The listing builds one solid part. Answer for the finished solid, in the listing's coordinates (mm). Face numbers are marked on the shaded views. A direction names the side the tool comes from. Round coordinates to 2 decimals unless told otherwise and drop trailing zeros. Write each loop counter-clockwise with the first axis right and the second up, starting at its lowest first coordinate (ties: lowest second). Pieces come first, ordered by that corner, then holes.
from build123d import *
from build123d.topology import SkipClean

# Parameters (mm, degrees)
SKETCH1_W                      = 4.2
SKETCH1_H                      = 2.4
F_0_8_0_8_DIAMETER_HOLE1_D     = 0.8
SKETCH6_R                      = 3.2
BOSS_EXTRUDE1_DEPTH            = 0.8
BOSS_EXTRUDE2_DEPTH            = 3
CUT_EXTRUDE1_DEPTH             = 2.2
BOSS_EXTRUDE3_DEPTH            = 2.2
BOSS_EXTRUDE4_DEPTH            = 0.8
BOSS_EXTRUDE5_START            = 1.6
SKETCH11_R                     = 2.4
BOSS_EXTRUDE5_DEPTH            = 1.6
SKETCH16_W                     = 7.2
SKETCH16_H                     = 1.6
F_3_2_3_2_DIAMETER_HOLE1_D     = 3.2
F_3_2_3_2_DIAMETER_HOLE1_DEPTH = 1.6


with BuildPart() as part:
    # Sketch1 → Revolve1 (revolve)
    with BuildSketch(Plane.XY):
        with Locations((-2.9, 1.2)):
            Rectangle(SKETCH1_W, SKETCH1_H)
    revolve(axis=Axis((-5, 0, 0), (1, 0, 0)))

    # Ø0.8 (0.8) Diameter Hole1 (through all)
    with Locations(Plane(origin=(-5, 0, -2.4), x_dir=(0, -1, 0), z_dir=(0, 0, -1))):
        with Locations((0, 0)):
            Hole(F_0_8_0_8_DIAMETER_HOLE1_D / 2)

    # Sketch6 → Boss-Extrude1 (add)
    with BuildSketch(Plane.ZY.offset(0.8)):
        Circle(SKETCH6_R)
    extrude(amount=-BOSS_EXTRUDE1_DEPTH)

    # Sketch7 → Boss-Extrude2 (add)
    with BuildSketch(Plane.ZY.offset(5)):
        with BuildLine():
            Line((-2.569046516, -0.4), (2.569046516, -0.4))
            ThreePointArc((2.569046516, -0.4), (0, -2.6), (-2.569046516, -0.4))
        make_face()
    extrude(amount=BOSS_EXTRUDE2_DEPTH)

    # Sketch8 → Cut-Extrude1 (cut)
    with SkipClean():  # the faces are left unmerged after this step: merging them gives an invalid solid
        with BuildSketch(Plane(origin=(-5, 0, 0), x_dir=(0, 0, -1), z_dir=(1, 0, 0))):
            with BuildLine():
                Line((2.569046516, -0.4), (2.366431913, -0.4))
                ThreePointArc((2.366431913, -0.4), (0, -2.4), (-2.366431913, -0.4))
                Line((-2.366431913, -0.4), (-2.569046516, -0.4))
                ThreePointArc((-2.569046516, -0.4), (0, -2.6), (2.569046516, -0.4))
            make_face()
        extrude(amount=-CUT_EXTRUDE1_DEPTH, mode=Mode.SUBTRACT)

    # Sketch9 → Boss-Extrude3 (add)
    with SkipClean():  # the faces are left unmerged after this step: merging them gives an invalid solid
        with BuildSketch(Plane.ZY.offset(5)):
            with BuildLine():
                Line((2.366431913, 0.4), (-2.366431913, 0.4))
                ThreePointArc((-2.366431913, 0.4), (0, 2.4), (2.366431913, 0.4))
            make_face()
        extrude(amount=BOSS_EXTRUDE3_DEPTH)

    # Sketch10 → Boss-Extrude4 (add)
    with SkipClean():  # the faces are left unmerged after this step: merging them gives an invalid solid
        with BuildSketch(Plane.ZY.offset(7.2)):
            with BuildLine():
                Line((2.569046516, 0.4), (-2.569046516, 0.4))
                ThreePointArc((-2.569046516, 0.4), (0, 2.6), (2.569046516, 0.4))
            make_face()
        extrude(amount=BOSS_EXTRUDE4_DEPTH)

    # Sketch11 → Boss-Extrude5 (add)
    with SkipClean():  # the faces are left unmerged after this step: merging them gives an invalid solid
        with BuildSketch(Plane(origin=(0, 0, 0), x_dir=(0, 0, -1), z_dir=(1, 0, 0)).offset(BOSS_EXTRUDE5_START)):
            with Locations(Location((0, 0, 0), (0, 0, 90))):
                Circle(SKETCH11_R)
        extrude(amount=-BOSS_EXTRUDE5_DEPTH)

    # Sketch16 → Cut-Revolve1 (revolve, cut)
    with SkipClean():  # the faces are left unmerged after this step: merging them gives an invalid solid
        with BuildSketch(Plane(origin=(0, 0, 0), x_dir=(-1, 0, 0), z_dir=(0, 0, -1)), mode=Mode.PRIVATE) as cut_revolve1_sk:
            with Locations((4.4, 0.8)):
                Rectangle(SKETCH16_W, SKETCH16_H)
        revolve(cut_revolve1_sk.sketch.rotate(Axis((-0.8, 0, 0), (-1, 0, 0)), 270), axis=Axis((-0.8, 0, 0), (-1, 0, 0)), mode=Mode.SUBTRACT)

    # Ø3.2 (3.2) Diameter Hole1
    with Locations(Plane(origin=(1.6, 0, 0), x_dir=(0, 0, -1), z_dir=(1, 0, 0))):
        with Locations((0, 0)):
            Hole(F_3_2_3_2_DIAMETER_HOLE1_D / 2, depth=F_3_2_3_2_DIAMETER_HOLE1_DEPTH)


solid = part.part
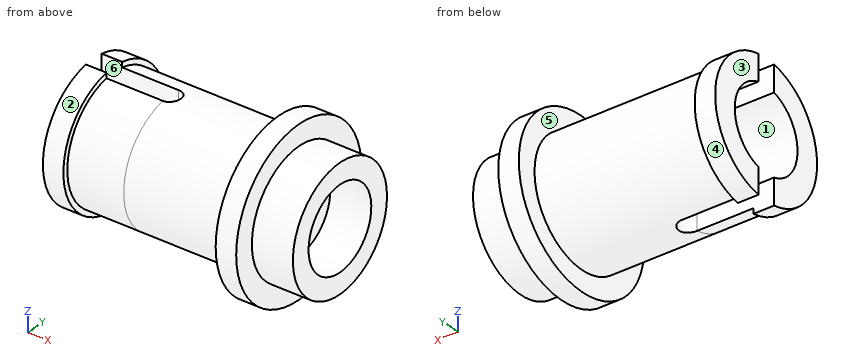
1. Given pin 1 (0.5 mm diameter, centred on x = -6.5, z = 2, fed in from +Y); pin 2 (1 mm diameter, centred on y = 0, z = -0.5, fed in from +X); pin 3 (0.8 mm diameter, centred on x = -6.5, z = 2, fed in from -Y), each flat-ended and moving along its own axis, determine where each tip first touches the part or whether it passes through.
Geometry says:
pin 1: stops at y = 1.64
pin 2: stops at x = 0
pin 3: stops at y = -1.79
2. Section A-A on x = -6 is taken. Determine the outline of the cut face in (y, z), plus the area to 3 significant figures.
Geometry says:
outline: (-0.4, -2.37) - (-0.4, -1.55) arc R1.6 cw to (-0.4, 1.55) - (-0.4, 2.37) arc R2.4 ccw to start; (0.4, -2.37) arc R2.4 ccw to (0.4, 2.37) - (0.4, 1.55) arc R1.6 cw to (0.4, -1.55) - close
area: 8.76 mm2
3. A tool of negligible diameter and unlimited length cuts with its end or side. For the marked faces 4, 5 and 6, from which of +Z, -Z, +X, -X, +Y, -Y can it reach the whole face along a straight path? Write none if from no direction.
Geometry says:
face 4: -X, +Y
face 5: none
face 6: +Z, -Z, -X
4. Section C-C on y = 0 is taken. Determine the outline of the cut face in (x, z).
Geometry says:
outline: (-4.6, -2.4) - (-0.8, -2.4) - (-0.8, -3.2) - (0, -3.2) - (0, -2.4) - (1.6, -2.4) - (1.6, -1.6) - (0, -1.6) - (0, 1.6) - (1.6, 1.6) - (1.6, 2.4) - (0, 2.4) - (0, 3.2) - (-0.8, 3.2) - (-0.8, 2.4) - (-4.6, 2.4) - (-4.6, 1.6) - (-0.8, 1.6) - (-0.8, -1.6) - (-4.6, -1.6) - close
5. Section D-D on z = 1 is taken. Determine the outline of the cut face in (x, y), plus the area to 3 significant figures.
Geometry says:
outline: (-8, -2.4) - (-7.2, -2.4) - (-7.2, -2.18) - (-0.8, -2.18) - (-0.8, -3.04) - (0, -3.04) - (0, -2.18) - (1.6, -2.18) - (1.6, -1.25) - (0, -1.25) - (0, 1.25) - (1.6, 1.25) - (1.6, 2.18) - (0, 2.18) - (0, 3.04) - (-0.8, 3.04) - (-0.8, 2.18) - (-7.2, 2.18) - (-7.2, 2.4) - (-8, 2.4) - (-8, 1.25) - (-0.8, 1.25) - (-0.8, -1.25) - (-8, -1.25) - close
area: 21.6 mm2
6. Section B-B on z = 0 is taken. Determine the outline of the cut face in (x, y).
Geometry says:
outline: (-8, -2.6) - (-7.2, -2.6) - (-7.2, -2.4) - (-0.8, -2.4) - (-0.8, -3.2) - (0, -3.2) - (0, -2.4) - (1.6, -2.4) - (1.6, -1.6) - (0, -1.6) - (0, 1.6) - (1.6, 1.6) - (1.6, 2.4) - (0, 2.4) - (0, 3.2) - (-0.8, 3.2) - (-0.8, 2.4) - (-7.2, 2.4) - (-7.2, 2.6) - (-8, 2.6) - (-8, 1.6) - (-0.8, 1.6) - (-0.8, -1.6) - (-8, -1.6) - close
7. Straight lines are drawn through the part: line 1 along Y through (x, z) = (-2.25, 0); line 2 along X through (y, z) = (-1.75, 1.75). For each, find the intervals that lie inside material, in ascending order.
Geometry says:
line 1: y = -2.4 to -1.6, 1.6 to 2.4
line 2: x = -8 to -7.2, -0.8 to 0
8. For a pull along Z with two mould halves and no side action, classify the marked faces 1, 2 and 3 as released by +Z, released by -Z, zero draft, split by the parting line, or undercut.
Geometry says:
face 1: undercut
face 2: split by the parting line
face 3: zero draft
